```python
from build123d import *

# Parameters (mm, degrees)
ESQUISSE2_R                  = 1.5
ENL_V_MAT_EXTRU_1_DEPTH      = 17
ENL_V_MAT_EXTRU_1_DEPTH_BACK = 17


with BuildPart() as part:
    # Esquisse1 → Révolution1 (revolve)
    with BuildSketch(Plane.XY):
        with BuildLine():
            Line((-170, 19.5), (-175, 19.5))
            Line((-175, 19.5), (-176, 18.5))
            Line((-176, 18.5), (-176, 3.5))
            Line((-176, 3.5), (-156, 3.5))
            Line((-156, 3.5), (-156, 15.35))
            Line((-156, 15.35), (-157, 16.35))
            Line((-157, 16.35), (-159, 16.35))
            Line((-159, 16.35), (-159, 14.6))
            ThreePointArc((-159, 14.6), (-159.146446609, 14.246446609), (-159.5, 14.1))
            Line((-159.5, 14.1), (-162.5, 14.1))
            ThreePointArc((-162.5, 14.1), (-162.853553391, 14.246446609), (-163, 14.6))
            Line((-163, 14.6), (-163, 16.35))
            Line((-163, 16.35), (-170, 16.35))
            Line((-170, 16.35), (-170, 19.5))
        make_face()
    revolve(axis=Axis((-170, 3.5, 0), (-1, 0, 0)))

    # Esquisse2 → Enlèv. mat.-Extru.1 (cut, two sides)
    with BuildSketch(Plane.XY) as enl_v_mat_extru_1_sk:
        with Locations((-166.5, 3.5)):
            Circle(ESQUISSE2_R)
    extrude(amount=ENL_V_MAT_EXTRU_1_DEPTH, mode=Mode.SUBTRACT)
    extrude(enl_v_mat_extru_1_sk.sketch, amount=-ENL_V_MAT_EXTRU_1_DEPTH_BACK, mode=Mode.SUBTRACT)


solid = part.part
```
Work out the finished part from the listing and answer in its coordinate system (mm). A direction names the side the tool comes from. Give positions to 0.01 mm unless a question says otherwise; leave off trailing zeros. Loops run counter-clockwise (first coordinate to the right, second up) from the corner with the lowest first, then second, coordinate; pieces in that order, holes last. Notation, with made-up numbers: M 37.5,84 L 51.5,84 A27 ccw 51.5,108 Z; hole C 40.5,21 d10. An arc over 180 degrees is marked long. One line per item, written item: value. Start each with the question number.
1. Find section B-B (z = 0). Give the vertices of the cut face in (x, y), and give its area (3 significant figures).
2. Determine the mould class of faces 4 (the face through (-161.02, 13.29, 4.06)), 5 (the face through (-176, 3, 0)), 6 (the face through (-156, 4, 0)) for opening direction X: released by +X, released by -X, zero draft, split by the parting line, or undercut.
3. Find section D-D (x = -166.5). Give the vertices of the cut face in (y, z).
4. Find section A-A (y = 3.5). Give the vertices of the cut face in (x, z), and give its area (3 significant figures).
5. Find the intervals of material crossed by probe 1 along X at (y, z) = (3.5, 0.5); probe 2 along Y at (x, z) = (-166.5, -7.25); probe 3 along Y at (x, z) = (-166.5, 6), in increasing order.
6. Which of the six approach directions +Z, -Z, +X, -X, +Y, -Y give full straight-line access (tool end or side, diameter ignored) to faces 1 (the face through (-172.535, 10.883, 14.195)), 2 (the face through (-166.549, 0.714, 12.544)), 3 (the face through (-159, 0, -11))?
7. Find section C-C (x = -158.25). Give the vertices of the cut face in (y, z).
8. Each of these flat-tipped pins is pushed along its axis until it touches: P1, Ø4, axis at x = -168.5, z = 3.5, coming from the +Y side; P2, Ø8, axis at x = -169, z = 6, coming from the -Y side; P3, Ø8, axis at x = -170, y = -2, coming from the -Z side. Where does it stop, or does it pass through?
Reported:
1. outline: M -176,-11.5 L -175,-12.5 L -170,-12.5 L -170,-9.35 L -163,-9.35 L -163,-7.6 A0.5 cw -162.5,-7.1 L -159.5,-7.1 A0.5 cw -159,-7.6 L -159,-9.35 L -157,-9.35 L -156,-8.35 L -156,15.35 L -157,16.35 L -159,16.35 L -159,14.6 A0.5 cw -159.5,14.1 L -162.5,14.1 A0.5 cw -163,14.6 L -163,16.35 L -170,16.35 L -170,19.5 L -175,19.5 L -176,18.5 Z; hole C -166.5,3.5 d3
1. area: 525 mm²
2. face 4: undercut
2. face 5: released by -X
2. face 6: released by +X
3. outline: M 2,-12.76 L 2,12.76 A12.85 ccw Z; M 5,-12.76 A12.85 ccw 5,12.76 Z
4. outline: M -176,-15 L -175,-16 L -170,-16 L -170,-12.85 L -168,-12.85 L -168,12.85 L -170,12.85 L -170,16 L -175,16 L -176,15 Z; M -165,-12.85 L -163,-12.85 L -163,-11.1 A0.5 cw -162.5,-10.6 L -159.5,-10.6 A0.5 cw -159,-11.1 L -159,-12.85 L -157,-12.85 L -156,-11.85 L -156,11.85 L -157,12.85 L -159,12.85 L -159,11.1 A0.5 cw -159.5,10.6 L -162.5,10.6 A0.5 cw -163,11.1 L -163,12.85 L -165,12.85 Z
4. area: 455 mm²
5. probe 1: x = -176 to -168, -165 to -156
5. probe 2: y = -7.11 to 2, 5 to 14.11
5. probe 3: y = -7.86 to 2, 5 to 14.86
6. face 1: +X, -X
6. face 2: +X
6. face 3: none
7. outline: C 3.5,0 d25.7
8. P1: stops at y = 19.35
8. P2: stops at y = -12.36
8. P3: stops at z = -15.93
